from build123d import *

# Parameters (mm, degrees)
F1_DEPTH = 7
F2_D     = 5.75


with BuildPart() as f1:
    # F0 (on Top) → F1 (new body)
    with BuildSketch(Plane.XY):
        Polygon((10.5, -50), (22.5, -50), (22.5, 50), (-14.5, 50), (-22.5, 50), (-22.5, 39), (-22.5, 16), (-22.5, 10), (-22.5, -47.25), (-10.5080957781, -47.25), (-10.6281967604, -6.0001864958), (10.3717142302, -5.9390441602), align=None)
        Polygon((-10.5, -50), (-10.5080957781, -47.25), (-22.5, -47.25), (-22.5, -50), align=None)
        Polygon((-22.5, 39), (-22.5, 50), (-50, 50.4175424576), (-50, -49.6404245496), (-22.5, -50), (-22.5, -47.25), (-22.5, 10), (-22.5, 16), align=None)
        Polygon((22.5, 50), (22.5, -50), (50, -49.6404245496), (50, 50.4175424576), align=None)
    extrude(amount=F1_DEPTH)

    # F2 (through all)
    with Locations(Plane(origin=(0, 0, 0), x_dir=(1, 0, 0), z_dir=(0, 0, -1))):
        with Locations((-10.5364832571, 37.5000529818), (10.4634277335, 37.4389106462)):
            Hole(F2_D / 2)


solid = f1.part
Build history of the part. All positions in model axes, mm. A direction names the side the tool comes from. Coordinates: 2 decimals unless noted, no trailing zeros. Write each loop counter-clockwise with the first axis right and the second up, starting at its lowest first coordinate (ties: lowest second). Pieces come first, ordered by that corner, then holes.
(1) Mould opens along X. For faces 1 (the flat face through (50, 0, 3)), 2 (the flat face through (0, 50, 3)), 3 (the flat face through (-1, 1, 0)) say: pulls with the +X half, pulls with the -X half, needs draft (parallel to the pull), parting line crosses it, or undercut.
(2) Pin check, flat tips, straight feed: pin 1 Ø4 at (x, y) = (20.5, -25.5) entering from -Z; pin 2 Ø3 at (x, z) = (-3.5, 4) entering from -Y; pin 3 Ø4 at (x, z) = (-34, 6) entering from -Y; pin 4 Ø1 at (x, z) = (11, 4) entering from +Y. Stop position of each tip, or through.
(3) Cut at B-B on x = -7. List the corners of the cut face in (y, z), and give its area (3 significant figures).
(4) Cut at A-A on z = 3. List the corners of the cut face in (x, y) (3 decimals).
(5) Drill centre lines: line 1 (X direction, y = -34, z = 2); line 2 (X direction, y = -26.5, z = 3.25); line 3 (Y direction, x = 2.5, z = 2.75). Where is each one in solid material? Low to high.
(6) 3-axis set-ups, long thin cutter, end or side, ignore diameter. For faces 4 (the flat face through (-1, 1, 7)), 5 (the cylindrical face through (-13.41, -37.45, 3.55)): which of +Z, -Z, +X, -X, +Y, -Y reach the whole face in a straight line?
Working result:
1. face 1: pulls with the +X half
1. face 2: undercut
1. face 3: needs draft
2. pin 1: stops at z = 0
2. pin 2: stops at y = -5.98
2. pin 3: stops at y = -49.88
2. pin 4: stops at y = 50
3. outline: (-5.99, 0) - (50, 0) - (50, 7) - (-5.99, 7) - close
3. area: 392 mm2
4. outline: (-50, -49.64) - (-22.5, -50) - (-10.5, -50) - (-10.508, -47.25) - (-10.528, -40.375) arc R2.875 cw to (-10.545, -34.625) - (-10.628, -6) - (10.372, -5.939) - (10.455, -34.564) arc R2.875 cw to (10.472, -40.314) - (10.5, -50) - (22.5, -50) - (50, -49.64) - (50, 50.418) - (22.5, 50) - (-22.5, 50) - (-50, 50.418) - close
5. line 1: x = -50 to -10.55, 10.45 to 50
5. line 2: x = -50 to -10.57, 10.43 to 50
5. line 3: y = -5.96 to 50
6. face 4: +Z, +X, -X, +Y, -Y
6. face 5: +Z, -Z
